from build123d import *

# Parameters (mm, degrees)
SKETCH1_R           = 47.5
BOSS_EXTRUDE1_DEPTH = 10
SKETCH2_W           = 8
SKETCH2_H           = 28
BOSS_EXTRUDE2_DEPTH = 35
SKETCH3_R           = 2.75
CUT_EXTRUDE1_DEPTH  = 70
SKETCH4_R           = 9
CUT_EXTRUDE2_DEPTH  = 5
CUT_EXTRUDE3_START  = -5
SKETCH5_R           = 9
CUT_EXTRUDE3_DEPTH  = 5
SKETCH6_R           = 7
CUT_EXTRUDE4_DEPTH  = 107.800272003
FILLET1_R           = 13
FILLET2_R           = 3
FILLET3_R           = 3
SKETCH7_W           = 10
SKETCH7_H           = 30
CUT_EXTRUDE5_DEPTH  = 76.7462871


with BuildPart() as part:
    # Sketch1 → Boss-Extrude1 (new body)
    with BuildSketch(Plane(origin=(0, 0, 0), x_dir=(1, 0, 0), z_dir=(0, 1, 0))):
        with Locations(Location((0, 0, 0), (0, 0, 270))):
            Circle(SKETCH1_R)
    extrude(amount=BOSS_EXTRUDE1_DEPTH)

    # Sketch2 → Boss-Extrude2 (add)
    with BuildSketch(Plane(origin=(0, 10, 0), x_dir=(1, 0, 0), z_dir=(0, 1, 0))):
        with Locations((-37.91, 0)):
            Rectangle(SKETCH2_W, SKETCH2_H)
        with Locations((37.91, 0)):
            Rectangle(SKETCH2_W, SKETCH2_H)
    extrude(amount=BOSS_EXTRUDE2_DEPTH)

    # Sketch3 → Cut-Extrude1 (cut)
    with BuildSketch(Plane(origin=(0, 10, 0), x_dir=(1, 0, 0), z_dir=(0, 1, 0))):
        with Locations(Location((-21.213203436, 21.213203436, 0), (0, 0, 270))):
            Circle(SKETCH3_R)
        with Locations(Location((21.213203436, 21.213203436, 0), (0, 0, 270))):
            Circle(SKETCH3_R)
        with Locations(Location((-21.213203436, -21.213203436, 0), (0, 0, 270))):
            Circle(SKETCH3_R)
    extrude(amount=-CUT_EXTRUDE1_DEPTH, mode=Mode.SUBTRACT)

    # Sketch4 → Cut-Extrude2 (cut)
    with BuildSketch(Plane.ZY.offset(41.91)):
        with Locations((0, 30)):
            Circle(SKETCH4_R)
    extrude(amount=-CUT_EXTRUDE2_DEPTH, mode=Mode.SUBTRACT)

    # Sketch5 → Cut-Extrude3 (cut)
    with BuildSketch(Plane(origin=(41.91, 0, 0), x_dir=(0, 0, -1), z_dir=(1, 0, 0)).offset(CUT_EXTRUDE3_START)):
        with Locations(Location((0, 30, 0), (0, 0, 180))):
            Circle(SKETCH5_R)
    extrude(amount=CUT_EXTRUDE3_DEPTH, mode=Mode.SUBTRACT)

    # Sketch6 → Cut-Extrude4 (cut, through all)
    with BuildSketch(Plane.ZY.offset(36.91)):
        with Locations(Location((0, 30, 0), (0, 0, 180))):
            Circle(SKETCH6_R)
    extrude(amount=-CUT_EXTRUDE4_DEPTH, mode=Mode.SUBTRACT)

    # Fillet1
    fillet1_edges = [part.edges().sort_by_distance(p)[0] for p in [
        (-37.91, 45, -14),
        (37.91, 45, -14),
        (37.91, 45, 14),
        (-37.91, 45, 14),
    ]]
    fillet(fillet1_edges, radius=FILLET1_R)

    # Fillet2
    fillet2_edges = [part.edges().sort_by_distance(p)[0] for p in [
        (33.91, 45, 0),
        (41.91, 45, 0),
        (41.91, 21, -14),
        (41.91, 21, 14),
        (41.91, 41.192388155, -10.192388155),
        (41.91, 41.192388155, 10.192388155),
        (33.91, 21, 14),
        (33.91, 21, -14),
        (33.91, 41.192388155, -10.192388155),
        (33.91, 41.192388155, 10.192388155),
        (-41.91, 45, 0),
        (-33.91, 45, 0),
        (-41.91, 21, 14),
        (-41.91, 21, -14),
        (-41.91, 41.192388155, 10.192388155),
        (-41.91, 41.192388155, -10.192388155),
        (-33.91, 21, -14),
        (-33.91, 21, 14),
        (-33.91, 41.192388155, 10.192388155),
        (-33.91, 41.192388155, -10.192388155),
    ]]
    fillet(fillet2_edges, radius=FILLET2_R)

    # Fillet3
    fillet3_edges = [part.edges().sort_by_distance(p)[0] for p in [
        (0, 10, -47.5),
    ]]
    fillet(fillet3_edges, radius=FILLET3_R)

    # Sketch7 → Cut-Extrude5 (cut, through all)
    with BuildSketch(Plane(origin=(0, 10, 0), x_dir=(1, 0, 0), z_dir=(0, 1, 0))):
        with Locations((-28.91, 0)):
            Rectangle(SKETCH7_W, SKETCH7_H)
        with Locations((28.91, 0)):
            Rectangle(SKETCH7_W, SKETCH7_H)
    extrude(amount=-CUT_EXTRUDE5_DEPTH, mode=Mode.SUBTRACT)


solid = part.part
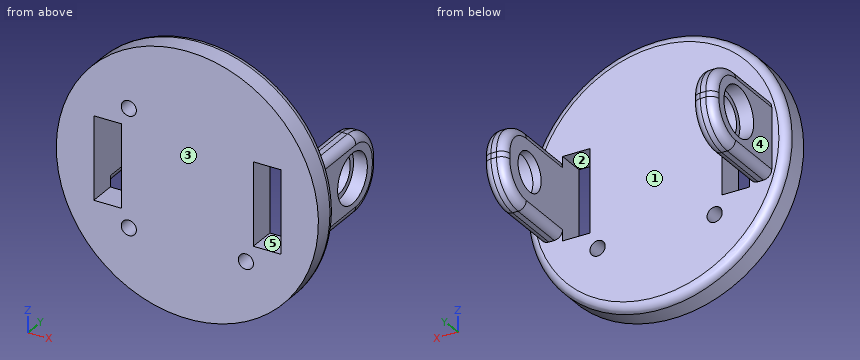
The listing builds one solid part. Answer for the finished solid, in the listing's coordinates (mm). Face numbers are marked on the shaded views. A direction names the side the tool comes from. Round coordinates to 2 decimals unless told otherwise and drop trailing zeros. Write each loop counter-clockwise with the first axis right and the second up, starting at its lowest first coordinate (ties: lowest second). Pieces come first, ordered by that corner, then holes. Notation, with made-up numbers: M 40,14.5 L 90,14.5 A24 ccw 90,24.5 Z; hole C 16,20.25 d5. An arc over 180 degrees is marked long. Write each question's results on one line, items separated by ' | '. Start each with the question number.
(1) Find the intervals of material crossed by line 1 (Y direction, x = 14, z = 23.5); line 2 (X direction, y = 5, z = -3); line 3 (Z direction, x = 38.3, y = 30), in increasing order.
(2) The part is cut by section A-A, the plane y = 30. Give the number of separate pieces and of enclosed holes in the cut face, and give its area (3 significant figures).
(3) For the marked faces 3, 4 and 5, determine the directions among +Z, -Z, +X, -X, +Y, -Y from which every point of the face is accessible in a straight line to the end or side of a thin tool.
(4) The part is cut by section B-B, the plane x = 0. Write down the section's boundary in (y, z), and give its area (3 significant figures).
(5) Each of these flat-tipped pins is pushed along its axis until it touches: P1, Ø6.5, axis at y = 33.5, z = 4.5, coming from the +X side; P2, Ø8, axis at x = 29.5, y = 5, coming from the -Z side; P3, Ø0.6, axis at x = 38.5, y = 23, coming from the +Z side. Where does it stop, or does it pass through?
(6) Determine the mould class of the marked faces 1 and 2 for opening direction Z: +Z half, -Z half, draft (parallel to the pull), parting line (faces both ways), or undercut.
Worked answers:
1) line 1: y = 0 to 10 | line 2: x = -47.41 to -33.91, -23.91 to 23.91, 33.91 to 47.41 | line 3: z = -14 to -9, 9 to 14
2) separate pieces: 4 | enclosed holes: 0 | area: 169 mm²
3) face 3: +Z, -Z, +X, -X, -Y | face 4: +Z, -Z, -X, +Y | face 5: +Y, -Y
4) outline: M 0,-47.5 L 7,-47.5 A3 ccw 10,-44.5 L 10,44.5 A3 ccw 7,47.5 L 0,47.5 Z | area: 946 mm²
5) P1: stops at x = 36.91 | P2: stops at z = -40.07 | P3: stops at z = 14
6) face 1: draft | face 2: undercut
